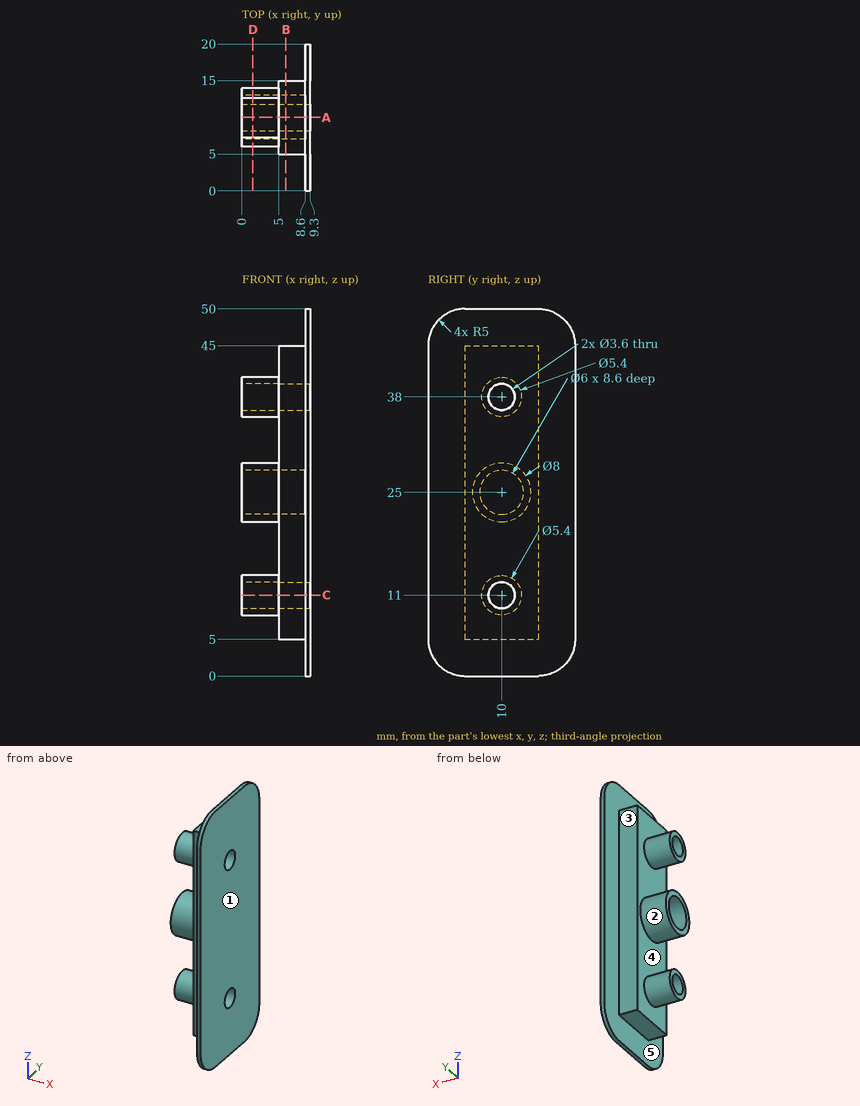
Job drawing, mm, ordinate dimensions from the low corner. One solid piece. A direction names the side the tool comes from. Coordinates: 2 decimals unless noted, no trailing zeros. Write each loop counter-clockwise with the first axis right and the second up, starting at its lowest first coordinate (ties: lowest second). Pieces come first, ordered by that corner, then holes. Notation, with made-up numbers: (76, 55.25) - (94, 55.25) arc R29 ccw to (94, 77.25) - close; hole circle Ø4 at (14.5, 33.25). An arc over 180 degrees is marked (long way). Use a Markdown table: item, result. Add a question column.
Item 1: Band-saw the part on B-B, the plane x = 6. Give the cut face in (y, z).
Item 2: Flat gauge pins, fed straight in: pin 1 (3 mm diameter, centred on x = 2, z = 28.5, fed in from +Y); pin 2 (1.8 mm diameter, centred on x = 6.5, y = 8, fed in from +Z); pin 3 (1.8 mm diameter, centred on x = 7, z = 32, fed in from +Y); pin 4 (2 mm diameter, centred on y = 10, z = 38, fed in from -X). Where does each tip first touch, or does it go through?
Item 3: Drill centre lines: L1, parallel to Z at x = 3.75, y = 9.75; L2, parallel to Z at x = 0.75, y = 10.5; L3, parallel to Y at x = 7, z = 11. Where is each one in solid material? Low to high. Write a range as from..to.
Item 4: Band-saw the part on C-C, the plane z = 11. Give the cut face in (x, y), and give its area (3 significant figures).
Item 5: 3-axis set-ups, long thin cutter, end or side, ignore diameter. For the marked faces 1, 2 and 3: which of +Z, -Z, +X, -X, +Y, -Y reach the whole face in a straight line?
Item 6: Band-saw the part on A-A, the plane y = 10. Give the number of separate pieces and of enclosed holes in the cut face, and give its area (3 significant figures).
Item 7: Mould opens along Z. For the marked faces 4 and 5 say: pulls with the +Z half, pulls with the -Z half, needs draft (parallel to the pull), parting line crosses it, or undercut.
Item 8: Band-saw the part on D-D, the plane x = 1.5. Give the cut face in (y, z), and give its area (3 significant figures).
Numbers:
| question | item | result |
|---|---|---|
| 1 | outline | (5, 5) - (15, 5) - (15, 45) - (5, 45) - close; hole circle Ø6 at (10, 25); hole circle Ø3.6 at (10, 11); hole circle Ø3.6 at (10, 38) |
| 2 | pin 1 | y = 13.46 |
| 2 | pin 2 | z = 45 |
| 2 | pin 3 | y = 15 |
| 2 | pin 4 | through |
| 3 | L1 | 8.31..9.22, 12.78..13.69, 21.01..22.01, 27.99..28.99, 35.31..36.22, 39.78..40.69 |
| 3 | L2 | 8.35..9.27, 12.73..13.65, 21.03..22.04, 27.96..28.97, 35.35..36.27, 39.73..40.65 |
| 3 | L3 | 5..8.2, 11.8..15 |
| 4 | outline | (0, 7.3) - (5, 7.3) - (5, 5) - (8.6, 5) - (8.6, 0) - (9.3, 0) - (9.3, 8.2) - (0, 8.2) - close; (0, 11.8) - (9.3, 11.8) - (9.3, 20) - (8.6, 20) - (8.6, 15) - (5, 15) - (5, 12.7) - (0, 12.7) - close |
| 4 | area | 43.5 mm2 |
| 5 | face 1 | +Z, -Z, +X, +Y, -Y |
| 5 | face 2 | -X |
| 5 | face 3 | +Z, -Z, -X, +Y |
| 6 | separate pieces | 3 |
| 6 | enclosed holes | 0 |
| 6 | area | 154 mm2 |
| 7 | face 4 | undercut |
| 7 | face 5 | needs draft |
| 8 | outline | circle Ø8 at (10, 25); circle Ø5.4 at (10, 11); circle Ø5.4 at (10, 38); hole circle Ø6 at (10, 25); hole circle Ø3.6 at (10, 11); hole circle Ø3.6 at (10, 38) |
| 8 | area | 47.4 mm2 |
